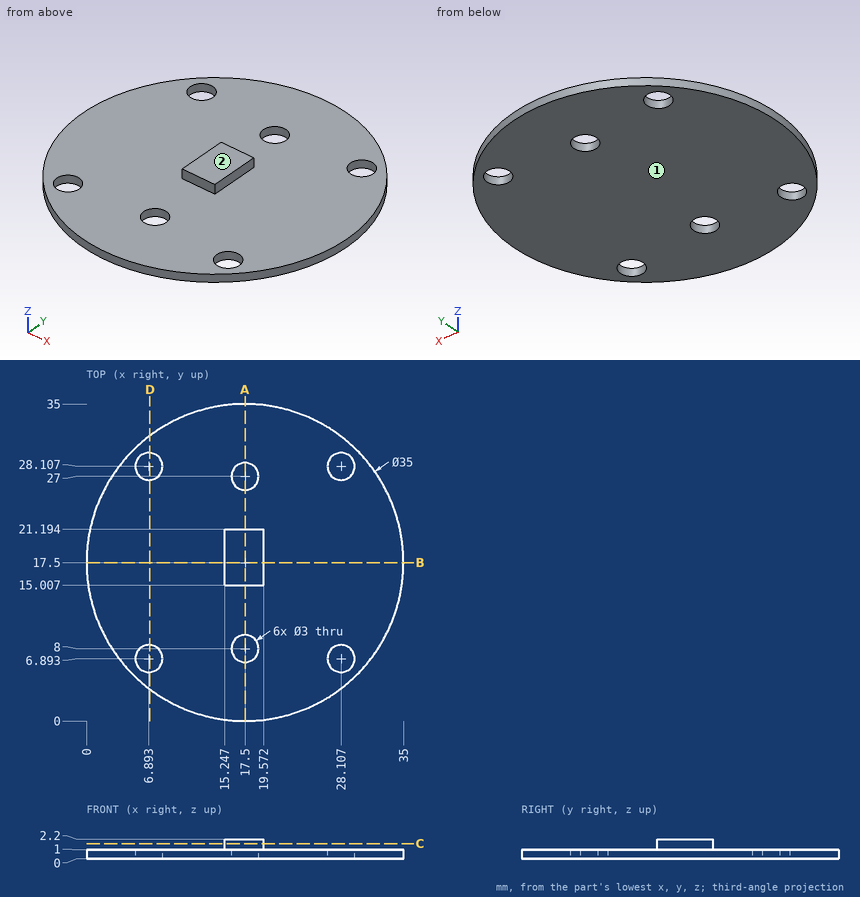
Input: dimensioned drawing with shaded views. Units: mm. Origin: part minimum x, y, z. Round coordinates to 2 decimals unless told otherwise and drop trailing zeros. Loops run counter-clockwise (first coordinate to the right, second up) from the corner with the lowest first, then second, coordinate; pieces in that order, holes last. Notation, with made-up numbers: M -37,-20.5 L 0,-20.5 A23 ccw 0,-0.5 Z; hole C 27.5,-23.75 d2. An arc over 180 degrees is marked long. Answer in a Markdown table with one row per item. Add a question column.
1. Ray query, probe 1 along Y at (x, z) = (17.5, 0.35); probe 2 along Y at (x, z) = (29, 0.5); probe 3 along Z at (x, y) = (32.5, 22.5). Return the intervals inside material, ascending.
2. Section C-C (z = 1.7). Output: boundary loops of the cut face in (x, y) (1 decimal).
3. Section B-B (y = 17.5). Output: boundary loops of the cut face in (x, z).
4. Contact query for flat-ended pins moving along their axis: pin 1 (5 mm diameter, centred on x = 17.5, y = 27, fed in from +Z); pin 2 (2.5 mm diameter, centred on x = 28.11, y = 6.89, fed in from +Z). Output: stop coordinate, or through.
5. Section D-D (x = 7). Output: boundary loops of the cut face in (y, z).
6. Mould query, pull axis Z, two halves, no side actions, for the marked faces 1 and 2. Classes: released by +Z, released by -Z, zero draft, split by the parting line, or undercut.
7. Section A-A (x = 17.5). Output: boundary loops of the cut face in (y, z) (1 decimal).
Values follow:
| question | item | result |
|---|---|---|
| 1 | probe 1 | 0 to 6.5, 9.5 to 25.5, 28.5 to 35 |
| 1 | probe 2 | 4.31 to 5.69, 8.1 to 26.9, 29.31 to 30.69 |
| 1 | probe 3 | 0 to 1 |
| 2 | outline | M 15.2,15 L 19.6,15 L 19.6,21.2 L 15.2,21.2 Z |
| 3 | outline | M 0,0 L 35,0 L 35,1 L 19.57,1 L 19.57,2.2 L 15.25,2.2 L 15.25,1 L 0,1 Z |
| 4 | pin 1 | z = 1 |
| 4 | pin 2 | through |
| 5 | outline | M 3.5,0 L 5.4,0 L 5.4,1 L 3.5,1 Z; M 8.39,0 L 26.61,0 L 26.61,1 L 8.39,1 Z; M 29.6,0 L 31.5,0 L 31.5,1 L 29.6,1 Z |
| 6 | face 1 | released by -Z |
| 6 | face 2 | released by +Z |
| 7 | outline | M 0,0 L 6.5,0 L 6.5,1 L 0,1 Z; M 9.5,0 L 25.5,0 L 25.5,1 L 21.2,1 L 21.2,2.2 L 15,2.2 L 15,1 L 9.5,1 Z; M 28.5,0 L 35,0 L 35,1 L 28.5,1 Z |
